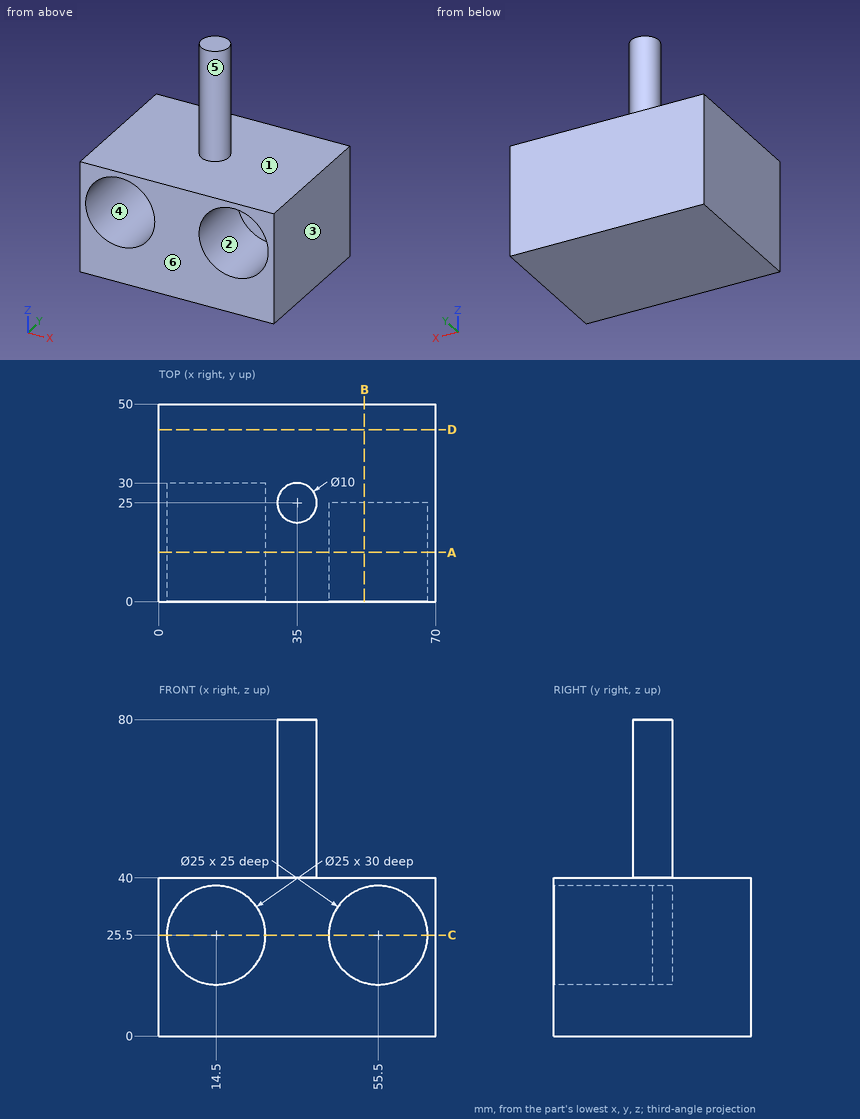
Design review of the part shown in the three views and the two pictorial views. Dimensions are in mm from the part's minimum x, y and z. A direction names the side the tool comes from. Give positions to 0.01 mm unless a question says otherwise; leave off trailing zeros. Write each loop counter-clockwise with the first axis right and the second up, starting at its lowest first coordinate (ties: lowest second). Pieces come first, ordered by that corner, then holes.
(1) Mouldability with a two-part tool opening along Z and no side actions: class the marked faces 1, 2, 3 and 4 as +Z half, -Z half, draft (parallel to the pull), parting line (faces both ways), or undercut.
Checked values:
face 1: +Z half
face 2: undercut
face 3: draft
face 4: undercut
(2) Add section A-A (y = 12.5). Give the boundary of the cut face in (x, z), and give its area (3 significant figures).
Checked values:
outline: (0, 0) - (70, 0) - (70, 40) - (0, 40) - close; hole circle Ø25 at (14.5, 25.5); hole circle Ø25 at (55.5, 25.5)
area: 1,820 mm2
(3) Add section D-D (y = 43.5). Give the boundary of the cut face in (x, z), and give its area (3 significant figures).
Checked values:
outline: (0, 0) - (70, 0) - (70, 40) - (0, 40) - close
area: 2,800 mm2
(4) Tool access review of the marked faces 5 and 6: name each direction out of +Z, -Z, +X, -X, +Y, -Y from which nothing blocks a thin tool from reaching the whole face with its end or side.
Checked values:
face 5: +Z
face 6: +Z, -Z, +X, -X, -Y
(5) Wall thickness on line 1 along Z through (x, y) = (55.5, 8.5); line 2 along X through (y, z) = (2.5, 15); line 3 along Z through (x, y) = (56.5, 30): over which ranges is each line inside the solid? List them lowest first.
Checked values:
line 1: z = 0 to 13, 38 to 40
line 2: x = 0 to 7.72, 21.28 to 48.72, 62.28 to 70
line 3: z = 0 to 40
(6) Add section B-B (x = 52). Give the boundary of the cut face in (y, z), and give its area (3 significant figures).
Checked values:
outline: (0, 0) - (50, 0) - (50, 40) - (0, 40) - (0, 37.5) - (25, 37.5) - (25, 13.5) - (0, 13.5) - close
area: 1,400 mm2
(7) Add section C-C (z = 25.5). Give the boundary of the cut face in (x, y).
Checked values:
outline: (0, 0) - (2, 0) - (2, 30) - (27, 30) - (27, 0) - (43, 0) - (43, 25) - (68, 25) - (68, 0) - (70, 0) - (70, 50) - (0, 50) - close
